from build123d import *

# Parameters (mm, degrees)
SKETCH1_R           = 8.5
BOSS_EXTRUDE1_DEPTH = 20
BOSS_EXTRUDE2_DEPTH = 5
SKETCH3_R           = 12.74933558
BOSS_EXTRUDE3_DEPTH = 30
SKETCH4_W           = 17.102448084
SKETCH4_H           = 17.762774264
BOSS_EXTRUDE4_DEPTH = 15
SKETCH5_R           = 6.477355188
SKETCH5_R_2         = 4.477355188
EXTRUDE_THIN1_DEPTH = 15


with BuildPart() as part:
    # Sketch1 → Boss-Extrude1 (new body)
    with BuildSketch(Plane(origin=(0, 0, 0), x_dir=(1, 0, 0), z_dir=(0, 1, 0))):
        with Locations(Location((0, 0, 0), (0, 0, 270))):
            Circle(SKETCH1_R)
    extrude(amount=-BOSS_EXTRUDE1_DEPTH)

    # Sketch2 → Boss-Extrude2 (add)
    with BuildSketch(Plane(origin=(0, 0, 0), x_dir=(1, 0, 0), z_dir=(0, 1, 0))):
        Polygon((0, 15), (-12.990381057, 7.5), (-12.990381057, -7.5), (0, -15), (12.990381057, -7.5), (12.990381057, 7.5), align=None)
    extrude(amount=BOSS_EXTRUDE2_DEPTH)

    # Sketch3 → Boss-Extrude3 (add)
    with BuildSketch(Plane(origin=(0, 5, 0), x_dir=(1, 0, 0), z_dir=(0, 1, 0))):
        with Locations(Location((0, 0, 0), (0, 0, 270))):
            Circle(SKETCH3_R)
    extrude(amount=BOSS_EXTRUDE3_DEPTH)

    # Sketch4 → Boss-Extrude4 (add)
    with BuildSketch(Plane(origin=(0, 35, 0), x_dir=(1, 0, 0), z_dir=(0, 1, 0))):
        Rectangle(SKETCH4_W, SKETCH4_H)
    extrude(amount=BOSS_EXTRUDE4_DEPTH)

    # Sketch5 → Extrude-Thin1 (add)
    with BuildSketch(Plane(origin=(8.551224042, 0, 0), x_dir=(0, 0, -1), z_dir=(1, 0, 0))):
        with Locations((0, 43.522644812)):
            Circle(SKETCH5_R)
        with Locations((0, 43.522644812)):
            Circle(SKETCH5_R_2, mode=Mode.SUBTRACT)
    extrude(amount=EXTRUDE_THIN1_DEPTH)


solid = part.part
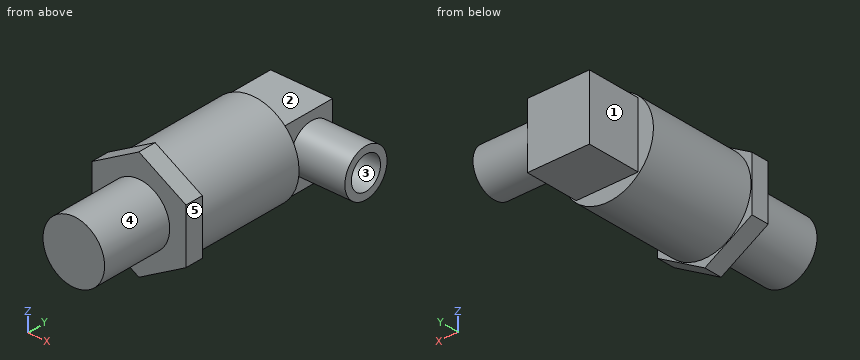
For this review, take the finished solid that the model builds, in its own axes (mm). Face numbers are marked on the shaded views. A direction names the side the tool comes from. Coordinates: 2 decimals unless noted, no trailing zeros. Loops run counter-clockwise (first coordinate to the right, second up) from the corner with the lowest first, then second, coordinate; pieces in that order, holes last. Notation, with made-up numbers: (-4.5, -34.75) - (22.5, -34.75) arc R17 ccw to (22.5, -23.75) - close; hole circle Ø3 at (2.25, -31.75). An arc over 180 degrees is marked (long way). Use a Markdown table: item, result. Add a question column.
Item 1: Insertion check: pin 1 Ø4.5 at (x, y) = (1.5, 45) entering from -Z; pin 2 Ø16.5 at (y, z) = (39, 0) entering from -X; pin 3 Ø8 at (y, z) = (-11, -3) entering from -X. Each pin has a flat end and moves straight along its axis. Give the tip position at first contact, or say it passes through.
Item 2: We need section B-B (z = 5.75). Give the boundary of the cut face in (x, y), and give its area (3 significant figures).
Item 3: Tool access review of the marked faces 1, 2, 3, 4 and 5: name each direction out of +Z, -Z, +X, -X, +Y, -Y from which nothing blocks a thin tool from reaching the whole face with its end or side.
Item 4: For line 1 (Y direction, x = 14.75, z = 0); line 2 (X direction, y = 45, z = -7.25); line 3 (Y direction, x = -3, z = 9.25), list the stretches that pass through material, from the lowest coordinate up.
Item 5: We need section D-D (y = -11.5). Give the boundary of the cut face in (x, z).
Item 6: We need section A-A (x = 10). Give the boundary of the cut face in (y, z), and give its area (3 significant figures).
Item 7: We need section C-C (x = -2). Give the boundary of the cut face in (y, z).
Results list:
| question | item | result |
|---|---|---|
| 1 | pin 1 | stops at z = -8.88 |
| 1 | pin 2 | stops at x = -12.75 |
| 1 | pin 3 | stops at x = -8.5 |
| 2 | outline | (-12.99, 0) - (-6.26, 0) - (-6.26, -20) - (6.26, -20) - (6.26, 0) - (12.99, 0) - (12.99, 5) - (11.38, 5) - (11.38, 35) - (8.55, 35) - (8.55, 40.54) - (23.55, 40.54) - (23.55, 46.5) - (8.55, 46.5) - (8.55, 50) - (-8.55, 50) - (-8.55, 35) - (-11.38, 35) - (-11.38, 5) - (-12.99, 5) - close |
| 2 | area | 1,410 mm^2 |
| 3 | face 1 | +Z, -Z, -X, +Y |
| 3 | face 2 | +Z, +X, -X, +Y |
| 3 | face 3 | +X |
| 3 | face 4 | -Y |
| 3 | face 5 | +Z, -Z, +X, -Y |
| 4 | line 1 | y = 37.05 to 39.05, 48 to 50 |
| 4 | line 2 | x = -8.55 to 8.55 |
| 4 | line 3 | y = 0 to 35 |
| 5 | outline | circle Ø17 at (0, 0) |
| 6 | outline | (0, -9.23) - (5, -9.23) - (5, -7.91) - (35, -7.91) - (35, 7.91) - (5, 7.91) - (5, 9.23) - (0, 9.23) - close; circle Ø12.95 at (43.52, 0); hole circle Ø8.95 at (43.52, 0) |
| 6 | area | 636 mm^2 |
| 7 | outline | (-20, -8.26) - (0, -8.26) - (0, -13.85) - (5, -13.85) - (5, -12.59) - (35, -12.59) - (35, -8.88) - (50, -8.88) - (50, 8.88) - (35, 8.88) - (35, 12.59) - (5, 12.59) - (5, 13.85) - (0, 13.85) - (0, 8.26) - (-20, 8.26) - close |
